```python
from build123d import *

# Parameters (mm, degrees)
SKETCH1_R               = 10
SKETCH1_R_2             = 2.6
BOSS_EXTRUDE1_DEPTH     = 25
BOSS_EXTRUDE2_START     = -5
SKETCH2_R               = 10
BOSS_EXTRUDE2_DEPTH     = 5
CUT_EXTRUDE1_DEPTH      = 29.722813233
CUT_EXTRUDE1_DEPTH_BACK = 29.722813233
SKETCH3_R               = 1.35
SKETCH6_R               = 10
SKETCH6_R_2             = 3.3734375
BOSS_EXTRUDE4_DEPTH     = 10
CUT_EXTRUDE2_DEPTH      = 38.74917233
CUT_EXTRUDE2_DEPTH_BACK = 38.74917233
SKETCH7_R               = 1.35
CUT_EXTRUDE3_DEPTH      = 38.74917233
CUT_EXTRUDE3_DEPTH_BACK = 38.74917233
SKETCH8_R               = 1.35
SKETCH5_R               = 10
BOSS_EXTRUDE3_DEPTH     = 5.56
CUT_EXTRUDE4_START      = -6.5
SKETCH9_R               = 3
CUT_EXTRUDE4_DEPTH      = 25.4
CUT_EXTRUDE5_START      = -6.5
SKETCH10_R              = 3
CUT_EXTRUDE5_DEPTH      = 25.4
CIRPATTERN1_COUNT       = 4


with BuildPart() as part:
    # Sketch1 → Boss-Extrude1 (new body)
    with BuildSketch(Plane.XY):
        Circle(SKETCH1_R)
        Circle(SKETCH1_R_2, mode=Mode.SUBTRACT)
    extrude(amount=BOSS_EXTRUDE1_DEPTH)

    # Sketch2 → Boss-Extrude2 (add)
    with BuildSketch(Plane.XY.offset(25).offset(BOSS_EXTRUDE2_START)):
        Circle(SKETCH2_R)
    extrude(amount=BOSS_EXTRUDE2_DEPTH)

    # Sketch3 → Cut-Extrude1 (cut, two sides: drawn at the far end of the back side and taken through both)
    with BuildSketch(Plane(origin=(0, 0, 0), x_dir=(1, 0, 0), z_dir=(0, 1, 0)).offset(-CUT_EXTRUDE1_DEPTH_BACK)):
        with Locations(Location((0, -10, 0), (0, 0, 270))):
            Circle(SKETCH3_R)
    extrude(amount=CUT_EXTRUDE1_DEPTH + CUT_EXTRUDE1_DEPTH_BACK, mode=Mode.SUBTRACT)

    # Sketch6 → Boss-Extrude4 (add)
    with BuildSketch(Plane.XY.offset(25)):
        Circle(SKETCH6_R)
        Circle(SKETCH6_R_2, mode=Mode.SUBTRACT)
    extrude(amount=BOSS_EXTRUDE4_DEPTH)

    # Sketch7 → Cut-Extrude2 (cut, two sides: drawn at the far end of the back side and taken through both)
    with BuildSketch(Plane(origin=(0, 0, 0), x_dir=(1, 0, 0), z_dir=(0, 1, 0)).offset(-CUT_EXTRUDE2_DEPTH_BACK)):
        with Locations(Location((0, -30, 0), (0, 0, 270))):
            Circle(SKETCH7_R)
    extrude(amount=CUT_EXTRUDE2_DEPTH + CUT_EXTRUDE2_DEPTH_BACK, mode=Mode.SUBTRACT)

    # Sketch8 → Cut-Extrude3 (cut, two sides: drawn at the far end of the back side and taken through both)
    with BuildSketch(Plane(origin=(0, 0, 0), x_dir=(0, 0, -1), z_dir=(1, 0, 0)).offset(-CUT_EXTRUDE3_DEPTH_BACK)):
        with Locations((-30, 0)):
            Circle(SKETCH8_R)
    extrude(amount=CUT_EXTRUDE3_DEPTH + CUT_EXTRUDE3_DEPTH_BACK, mode=Mode.SUBTRACT)

    # Sketch5 → Boss-Extrude3 (add)
    with BuildSketch(Plane.XY.offset(35)):
        Circle(SKETCH5_R)
        Polygon((3.204293994, -5.55), (6.408587988, 0), (3.204293994, 5.55), (-3.204293994, 5.55), (-6.408587988, 0), (-3.204293994, -5.55), align=None, mode=Mode.SUBTRACT)
    extrude(amount=BOSS_EXTRUDE3_DEPTH)

    # Sketch9 → Cut-Extrude4 (cut)
    with BuildSketch(Plane(origin=(0, 0, 0), x_dir=(1, 0, 0), z_dir=(0, 1, 0)).offset(CUT_EXTRUDE4_START)):
        with Locations(Location((0, -10, 0), (0, 0, 270))):
            Circle(SKETCH9_R)
    cut_extrude4 = extrude(amount=-CUT_EXTRUDE4_DEPTH, mode=Mode.SUBTRACT)

    # Mirror1: Cut-Extrude4 across plane
    add(cut_extrude4.mirror(Plane.ZX), mode=Mode.SUBTRACT)

    # Sketch10 → Cut-Extrude5 (cut)
    with BuildSketch(Plane(origin=(0, 0, 0), x_dir=(1, 0, 0), z_dir=(0, 1, 0)).offset(CUT_EXTRUDE5_START)):
        with Locations(Location((0, -30, 0), (0, 0, 270))):
            Circle(SKETCH10_R)
    cut_extrude5 = extrude(amount=-CUT_EXTRUDE5_DEPTH, mode=Mode.SUBTRACT)

    # CirPattern1: Cut-Extrude5 ×4 about axis
    cirpattern1_axis = Axis((0, 0, 0), (0, 0, 1))
    for i in range(1, CIRPATTERN1_COUNT):
        add(cut_extrude5.rotate(cirpattern1_axis, i * 360 / CIRPATTERN1_COUNT), mode=Mode.SUBTRACT)


solid = part.part
```
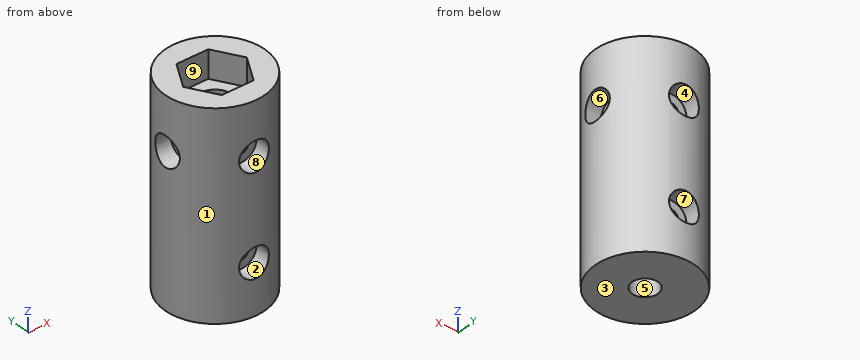
The listing builds one solid part. Answer for the finished solid, in the listing's coordinates (mm). Face numbers are marked on the shaded views. A direction names the side the tool comes from. Coordinates: 2 decimals unless noted, no trailing zeros. Loops run counter-clockwise (first coordinate to the right, second up) from the corner with the lowest first, then second, coordinate; pieces in that order, holes last. Notation, with made-up numbers: (63, -38.5) - (115, -38.5) arc R28 ccw to (115, -17.5) - close; hole circle Ø3 at (21, -30). An arc over 180 degrees is marked (long way). Write item = value, one per line.
1) Section D-D (x = 0) is taken. Count the separate pieces of the cut face and the enclosed holes in it, plus the area to 3 significant figures.
Responses:
separate_pieces = 5
enclosed_holes = 0
area = 456 mm^2
2) Section B-B (y = 8) is taken. Determine the outline of the cut face in (x, z), plus the area to 3 significant figures.
Responses:
outline = (-6, 0) - (6, 0) - (6, 40.56) - (-6, 40.56) - close; hole circle Ø6 at (0, 10); hole circle Ø6 at (0, 30)
area = 430 mm^2
3) Each of these flat-tipped pins is pushed along its axis until it touches: P1, Ø2.5, axis at x = 0, z = 10, coming from the -Y side; P2, Ø1.8, axis at y = -1, z = 30, coming from the +X side; P3, Ø3, axis at x = 0, z = 30, coming from the +Y side; P4, Ø1.5, axis at x = 4, z = 17.5, coming from the -Y side. Where does it stop, or does it pass through?
Responses:
P1 = through
P2 = 6.5
P3 = 6.5
P4 = -9.46
4) Find the intervals of material crossed by line 1 along Z through (x, y) = (0, -7.8); line 2 along X through (y, z) = (0, 15); line 3 along Z through (x, y) = (1.5, -4), in increasing order.
Responses:
line_1 = 0 to 7, 13 to 27, 33 to 40.56
line_2 = -10 to -2.6, 2.6 to 10
line_3 = 0 to 35
5) Section A-A (z = 10) is taken. Determine the outline of the cut face in (x, y), plus the area to 3 significant figures.
Responses:
outline = (-3, -9.54) - (-3, -6.5) - (-1.35, -6.5) - (-1.35, -2.22) arc R2.6 cw to (-1.35, 2.22) - (-1.35, 6.5) - (-3, 6.5) - (-3, 9.54) arc R10 ccw to start; (1.35, -6.5) - (3, -6.5) - (3, -9.54) arc R10 ccw to (3, 9.54) - (3, 6.5) - (1.35, 6.5) - (1.35, 2.22) arc R2.6 cw to (1.35, -2.22) - close
area = 231 mm^2
6) Section C-C (x = 4) is taken. Determine the outline of the cut face in (y, z).
Responses:
outline = (-9.17, 0) - (9.17, 0) - (9.17, 40.56) - (4.17, 40.56) - (4.17, 35) - (-4.17, 35) - (-4.17, 40.56) - (-9.17, 40.56) - close; hole circle Ø2.7 at (0, 30)
7) Determine the mould class of the marked faces 1, 2, 3 and 4 for opening direction X: pulls with the +X half, pulls with the -X half, needs draft (parallel to the pull), parting line crosses it, or undercut.
Responses:
face_1 = parting line crosses it
face_2 = undercut
face_3 = needs draft
face_4 = undercut
8) Which of the six approach directions +Z, -Z, +X, -X, +Y, -Y give full straight-line access (tool end or side, diameter ignored) to the marked faces 5, 6, 7, 8 and 9?
Responses:
face_5 = -Z
face_6 = +X
face_7 = +Y
face_8 = -Y
face_9 = +Z
